The model under review builds one solid part; all positions refer to its coordinate system, in mm. Coordinates: 2 decimals unless noted, no trailing zeros. Loops run counter-clockwise (first coordinate to the right, second up) from the corner with the lowest first, then second, coordinate; pieces in that order, holes last. Notation, with made-up numbers: (36, -22) - (89, -22) arc R22 cw to (89, -8) - close; hole circle Ø3 at (83.5, 33.5). An arc over 180 degrees is marked (long way). Use a Markdown table: item, result. Add a question column.
1) To check wall thickness, follow L1, parallel to Y at x = -23.75, z = 0.8; L2, parallel to Y at x = -11.25, z = 1.6; L3, parallel to X at y = 6.25, z = 1.35. State the ranges of each line that lie inside material, in increasing order. Write a range as [from, to].
2) Add section B-B, the plane y = 19. Give the boundary of the cut face in (x, z), and give its area (3 significant figures).
3) Add section C-C, the plane z = 1.6. Give the number of separate pieces and of enclosed holes in the cut face, and give its area (3 significant figures).
4) Add section A-A, the plane x = -4.75. Give the boundary of the cut face in (y, z).
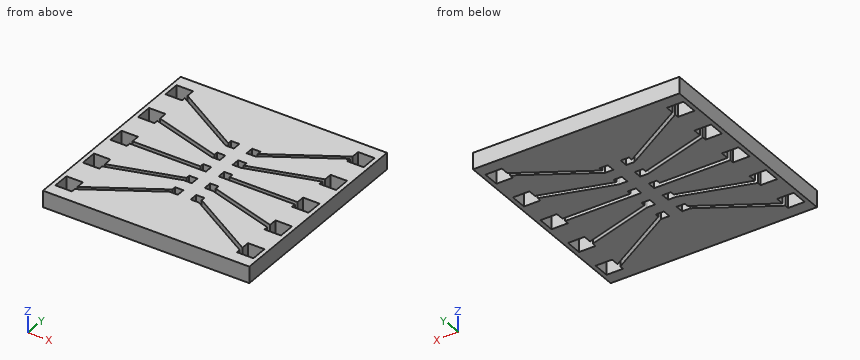
```python
from build123d import *

# Parameters (mm, degrees)
F0_W     = 25
F0_H     = 25
F1_DEPTH = 2
F3_DEPTH = 2


# Not quite as in the source:
# - a feature names something its author has since deleted; it is built from what else it names


with BuildPart() as f1:
    # F0 (on Top) → F1 (new body)
    with BuildSketch(Plane.XY):
        with Locations((-12.5, 12.5)):
            Rectangle(F0_W, F0_H)
    extrude(amount=F1_DEPTH)

    # F2 (on face) → F3 (cut)
    with BuildSketch(Plane.XY.offset(2)):
        Polygon((-13.275, 15.54), (-14.275, 15.54), (-14.275, 15.04), (-22.5, 17.5), (-22.5, 18.5), (-24.5, 18.5), (-24.5, 16.5), (-22.5, 16.5), (-22.5, 17), (-14.275, 14.54), (-13.275, 14.54), align=None)
        Polygon((-13.275, 18.08), (-14.275, 18.08), (-14.275, 17.58), (-22.5, 22.5), (-22.5, 23.5), (-24.5, 23.5), (-24.5, 21.5), (-22.5, 21.5), (-22.5, 22), (-14.275, 17.08), (-13.275, 17.08), align=None)
        Polygon((-13.275, 13), (-14.275, 13), (-14.275, 12.5), (-22.5, 12.5), (-22.5, 13.5), (-24.5, 13.5), (-24.5, 11.5), (-22.5, 11.5), (-22.5, 12), (-14.275, 12), (-13.275, 12), align=None)
        Polygon((-13.275, 10.46), (-14.275, 10.46), (-14.275, 9.96), (-22.5, 7.5), (-22.5, 8.5), (-24.5, 8.5), (-24.5, 6.5), (-22.5, 6.5), (-22.5, 7), (-14.275, 9.46), (-13.275, 9.46), align=None)
        Polygon((-13.275, 7.92), (-14.275, 7.92), (-14.275, 7.42), (-22.5, 2.5), (-22.5, 3.5), (-24.5, 3.5), (-24.5, 1.5), (-22.5, 1.5), (-22.5, 2), (-14.275, 6.92), (-13.275, 6.92), align=None)
        Polygon((-10.725, 6.92), (-2.5, 2), (-2.5, 1.5), (-0.5, 1.5), (-0.5, 3.5), (-2.5, 3.5), (-2.5, 2.5), (-10.725, 7.42), (-10.725, 7.92), (-11.725, 7.92), (-11.725, 6.92), align=None)
        Polygon((-11.725, 12), (-10.725, 12), (-2.5, 12), (-2.5, 11.5), (-0.5, 11.5), (-0.5, 13.5), (-2.5, 13.5), (-2.5, 12.5), (-10.725, 12.5), (-10.725, 13), (-11.725, 13), align=None)
        Polygon((-11.725, 14.54), (-10.725, 14.54), (-2.5, 17), (-2.5, 16.5), (-0.5, 16.5), (-0.5, 18.5), (-2.5, 18.5), (-2.5, 17.5), (-10.725, 15.04), (-10.725, 15.54), (-11.725, 15.54), align=None)
        Polygon((-10.725, 17.58), (-10.725, 18.08), (-11.725, 18.08), (-11.725, 17.08), (-10.725, 17.08), (-2.5, 22), (-2.5, 21.5), (-0.5, 21.5), (-0.5, 23.5), (-2.5, 23.5), (-2.5, 22.5), align=None)
        Polygon((-10.725, 9.96), (-10.725, 10.46), (-11.725, 10.46), (-11.725, 9.46), (-10.725, 9.46), (-2.5, 7), (-2.5, 6.5), (-0.5, 6.5), (-0.5, 8.5), (-2.5, 8.5), (-2.5, 7.5), align=None)
    extrude(amount=-F3_DEPTH, mode=Mode.SUBTRACT)


solid = f1.part
```
From the geometry:
| question | item | result |
|---|---|---|
| 1 | L1 | y = [0, 1.5], [3.5, 6.5], [8.5, 11.5], [13.5, 16.5], [18.5, 21.5], [23.5, 25] |
| 1 | L2 | y = [0, 6.92], [7.92, 9.46], [10.46, 12], [13, 14.54], [15.54, 17.08], [18.08, 25] |
| 1 | L3 | x = [-25, -16.23], [-15.4, -9.6], [-8.77, 0] |
| 2 | outline | (-25, 0) - (-17.48, 0) - (-17.48, 2) - (-25, 2) - close; (-16.65, 0) - (-8.35, 0) - (-8.35, 2) - (-16.65, 2) - close; (-7.52, 0) - (0, 0) - (0, 2) - (-7.52, 2) - close |
| 2 | area | 46.7 mm^2 |
| 3 | separate pieces | 1 |
| 3 | enclosed holes | 10 |
| 3 | area | 534 mm^2 |
| 4 | outline | (0, 0) - (3.35, 0) - (3.35, 2) - (0, 2) - close; (3.85, 0) - (7.67, 0) - (7.67, 2) - (3.85, 2) - close; (8.17, 0) - (12, 0) - (12, 2) - (8.17, 2) - close; (12.5, 0) - (16.33, 0) - (16.33, 2) - (12.5, 2) - close; (16.83, 0) - (20.65, 0) - (20.65, 2) - (16.83, 2) - close; (21.15, 0) - (25, 0) - (25, 2) - (21.15, 2) - close |
